Check sheet for the drawn part. Datum: minimum x, y, z corner. Units: mm. A direction names the side the tool comes from. Give positions to 0.01 mm unless a question says otherwise; leave off trailing zeros. Loops run counter-clockwise (first coordinate to the right, second up) from the corner with the lowest first, then second, coordinate; pieces in that order, holes last. Notation, with made-up numbers: (-27.75, 6) - (24.25, 6) arc R16 cw to (24.25, 30) - close; hole circle Ø7 at (26, 31.25). An arc over 180 degrees is marked (long way). Use one line per item in the form item = value.
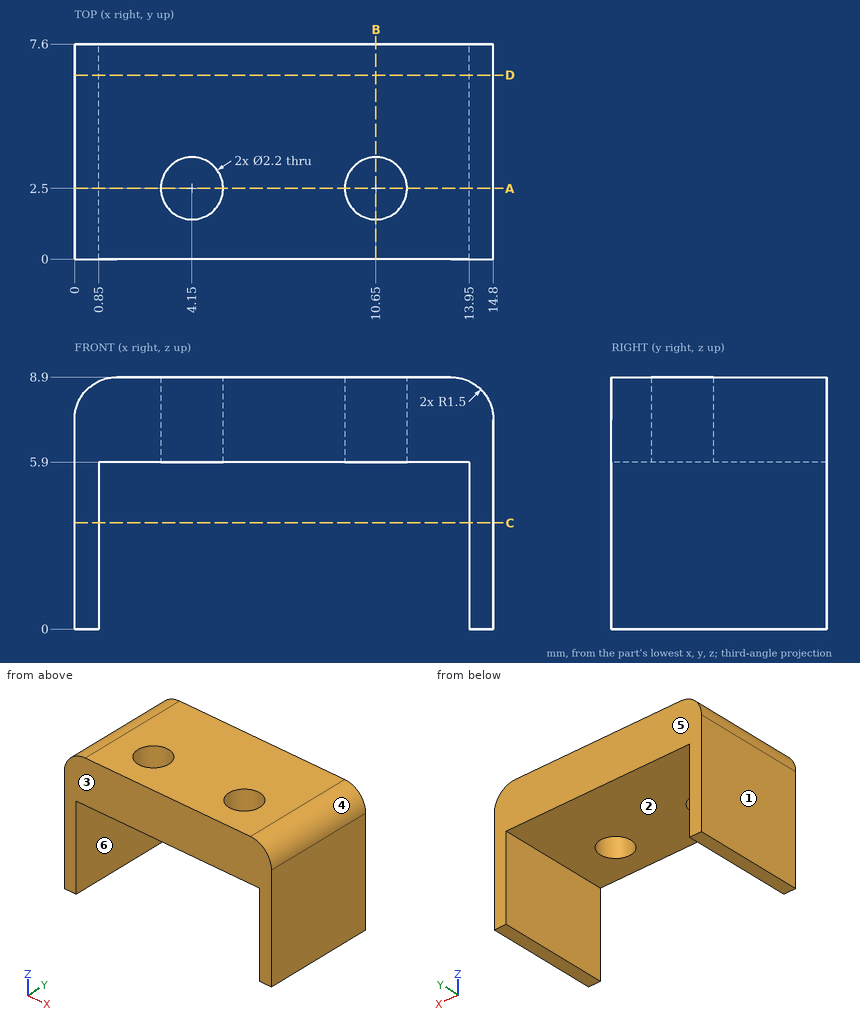
Item 1: Access from +Z, -Z, +X, -X, +Y, -Y to the whole of each face (thin tool, end or side, straight path). Record for the marked faces 5 and 6.
Answer block:
face_5 = +Z, -Z, +X, -X, +Y
face_6 = -Z, +Y, -Y
Item 2: Thickness scan on L1, parallel to Y at x = 10.65, z = 7.95; L2, parallel to X at y = 6.5, z = 2; L3, parallel to Z at x = 4.25, y = 5. Record the ranges inside material, lowest first.
Answer block:
L1 = 0 to 1.4, 3.6 to 7.6
L2 = 0 to 0.85, 13.95 to 14.8
L3 = 5.9 to 8.9
Item 3: Section check B-B on x = 10.65. Record the boundary of the cut face in (y, z).
Answer block:
outline = (0, 5.9) - (1.4, 5.9) - (1.4, 8.9) - (0, 8.9) - close; (3.6, 5.9) - (7.6, 5.9) - (7.6, 8.9) - (3.6, 8.9) - close
Item 4: Section check D-D on y = 6.5. Record the boundary of the cut face in (x, z).
Answer block:
outline = (0, 0) - (0.85, 0) - (0.85, 5.9) - (13.95, 5.9) - (13.95, 0) - (14.8, 0) - (14.8, 7.4) arc R1.5 ccw to (13.3, 8.9) - (1.5, 8.9) arc R1.5 ccw to (0, 7.4) - close
Item 5: Section check C-C on z = 3.75. Record the boundary of the cut face in (x, y), then the cut area to 3 significant figures.
Answer block:
outline = (0, 0) - (0.85, 0) - (0.85, 7.6) - (0, 7.6) - close; (13.95, 0) - (14.8, 0) - (14.8, 7.6) - (13.95, 7.6) - close
area = 12.9 mm2
Item 6: Section check A-A on y = 2.5. Record the boundary of the cut face in (x, z).
Answer block:
outline = (0, 0) - (0.85, 0) - (0.85, 5.9) - (3.05, 5.9) - (3.05, 8.9) - (1.5, 8.9) arc R1.5 ccw to (0, 7.4) - close; (5.25, 5.9) - (9.55, 5.9) - (9.55, 8.9) - (5.25, 8.9) - close; (11.75, 5.9) - (13.95, 5.9) - (13.95, 0) - (14.8, 0) - (14.8, 7.4) arc R1.5 ccw to (13.3, 8.9) - (11.75, 8.9) - close
Item 7: Mould release check, pull along X, two halves, no side actions. Record for the marked faces 1, 2, 3 and 4: released by +X, released by -X, zero draft, split by the parting line, or undercut.
Answer block:
face_1 = released by -X
face_2 = undercut
face_3 = zero draft
face_4 = released by +X
Item 8: Gauge pin test, flat ends, axial feed: P1, Ø4, axis at y = 3, z = 6, coming from the -X side; P2, Ø4, axis at x = 9, y = 2, coming from the -Z side; P3, Ø2, axis at x = 4.15, y = 2.5, coming from the -Z side. Record the tip position at first contact, or that the pin passes through.
Answer block:
P1 = 0
P2 = 5.9
P3 = through
